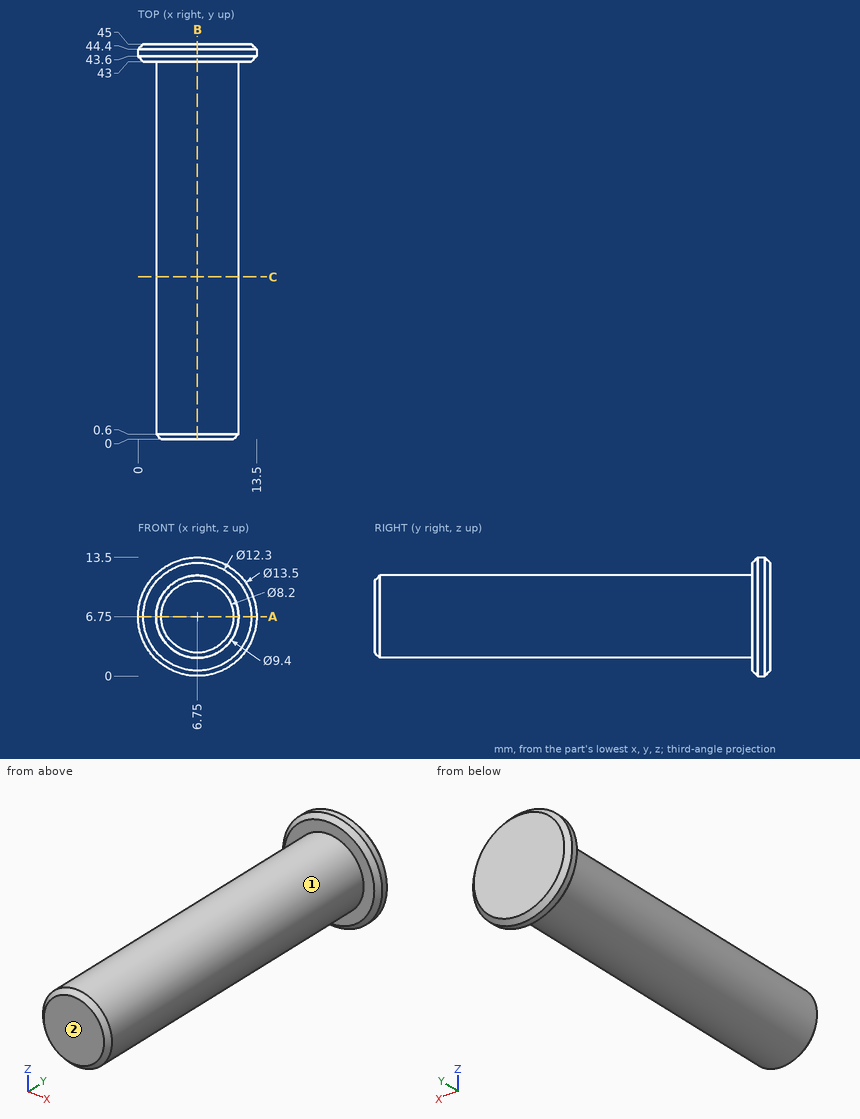
Check sheet for the drawn part. Datum: minimum x, y, z corner. Units: mm. A direction names the side the tool comes from. Coordinates: 2 decimals unless noted, no trailing zeros. Write each loop counter-clockwise with the first axis right and the second up, starting at its lowest first coordinate (ties: lowest second). Pieces come first, ordered by that corner, then holes. Notation, with made-up numbers: M 72,12.5 L 109,12.5 A20 cw 109,35.5 Z; hole C -28,22 d8. An arc over 180 degrees is marked long. One line per item, written item: value.
Item 1: Section check C-C, the plane y = 18.5. Record the boundary of the cut face in (x, z), plus the area to 3 significant figures.
Check sheet entries:
outline: C 6.75,6.75 d9.4
area: 69.4 mm^2
Item 2: Section check A-A, the plane z = 6.75. Record the boundary of the cut face in (x, y), plus the area to 3 significant figures.
Check sheet entries:
outline: M 0,43.6 L 0.6,43 L 2.05,43 L 2.05,0.6 L 2.65,0 L 10.85,0 L 11.45,0.6 L 11.45,43 L 12.9,43 L 13.5,43.6 L 13.5,44.4 L 12.9,45 L 0.6,45 L 0,44.4 Z
area: 430 mm^2
Item 3: Section check B-B, the plane x = 6.75. Record the boundary of the cut face in (y, z).
Check sheet entries:
outline: M 0,2.65 L 0.6,2.05 L 43,2.05 L 43,0.6 L 43.6,0 L 44.4,0 L 45,0.6 L 45,12.9 L 44.4,13.5 L 43.6,13.5 L 43,12.9 L 43,11.45 L 0.6,11.45 L 0,10.85 Z
Item 4: Gauge pin test, flat ends, axial feed: pin 1 Ø4 at (y, z) = (34.5, 11.5) entering from +X; pin 2 Ø1.5 at (x, z) = (4.5, 12) entering from -Y. Record the tip position at first contact, or that the pin passes through.
Check sheet entries:
pin 1: stops at x = 10.56
pin 2: stops at y = 43
Item 5: Scan lines: line 1 along Y through (x, z) = (2.75, 2.75); line 2 along X through (y, z) = (26.5, 6.75); line 3 along X through (y, z) = (36.5, 5.5). Record each from-to range of solid material in increasing order.
Check sheet entries:
line 1: y = 43 to 45
line 2: x = 2.05 to 11.45
line 3: x = 2.22 to 11.28
Item 6: Access from +Z, -Z, +X, -X, +Y, -Y to the whole of each face (thin tool, end or side, straight path). Record for the marked faces 1 and 2.
Check sheet entries:
face 1: -Y
face 2: +Z, -Z, +X, -X, -Y
